Answer from the drawing. Dimensions are ordinates in mm from the lowest x, y and z of the part. A direction names the side the tool comes from. Coordinates: 2 decimals unless noted, no trailing zeros. Write each loop counter-clockwise with the first axis right and the second up, starting at its lowest first coordinate (ties: lowest second). Pieces come first, ordered by that corner, then holes. Notation, with made-up numbers: (72, -27.5) -> (127, -27.5) arc R14 cw to (127, -1.5) -> close; hole circle Ø5 at (-4.75, 2). An arc over 180 degrees is marked (long way). Answer as a JSON object with one key per item and string values. Group by question number.
(1) Flat-ended cylindrical pins translate along their axes: P1, Ø4.5, axis at y = 5, z = 5, coming from the -X side; P2, Ø4.5, axis at x = 23.5, z = 5.5, coming from the -Y side; P3, Ø3, axis at x = 20.5, z = 7, coming from the -Y side. Find the tip coordinate at first contact, or state that the pin passes through.
(2) Which of the six approach directions +Z, -Z, +X, -X, +Y, -Y give full straight-line access (tool end or side, diameter ignored) to the marked faces 1, 2, 3, 4 and 5?
(3) Find section D-D (x = 6.25). Give the vertices of the cut face in (y, z).
(4) Straight lines are drawn through the part: L1, parallel to Y at x = 43.75, z = 2; L2, parallel to X at y = 30.5, z = 1; L3, parallel to X at y = 68.75, z = 4. For each, find the intervals that lie inside material, in ascending order.
(5) Find section C-C (y = 15). Give the vertices of the cut face in (x, z).
(6) Find section B-B (y = 31.25). Give the vertices of the cut face in (x, z).
(7) Find section A-A (x = 24.5). Give the vertices of the cut face in (y, z).
(8) For a pull along Y with two mould halves and no side action, classify the marked faces 6, 7, 8 and 9 as +Y half, -Y half, draft (parallel to the pull), parting line (faces both ways), or undercut.
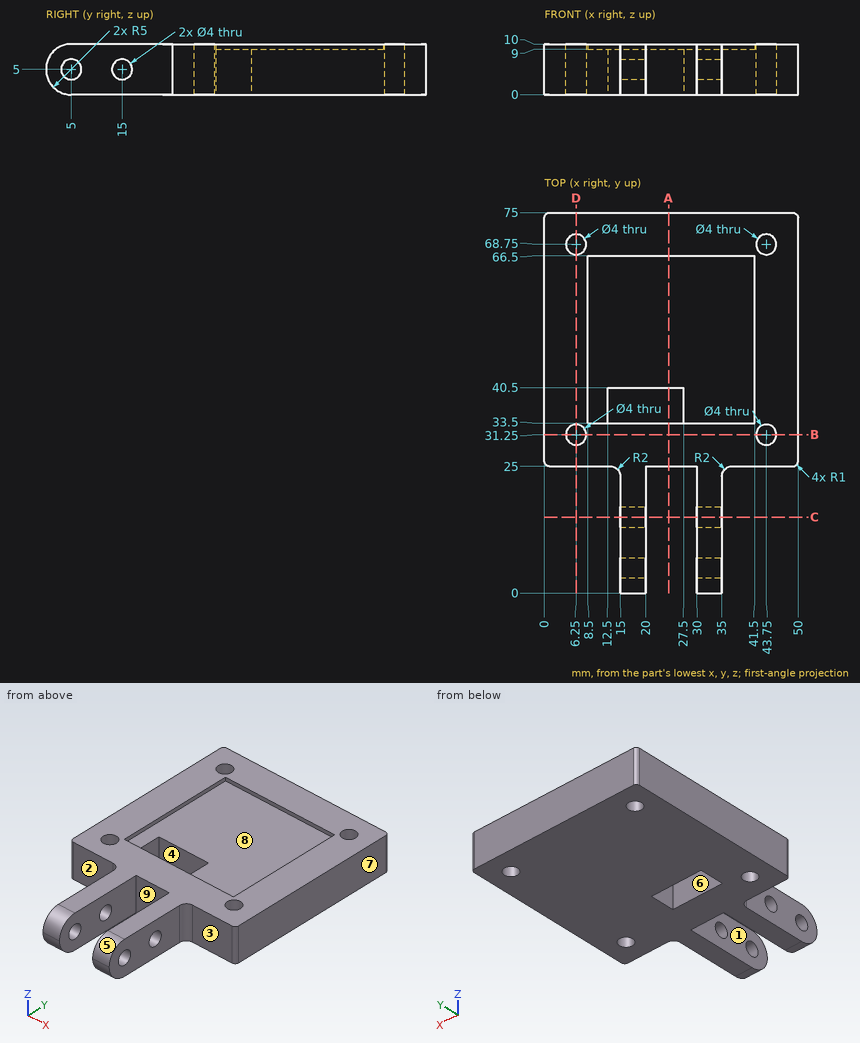
Results below:
{
 "1": {"P1": "stops at x = 15", "P2": "stops at y = 25", "P3": "stops at y = 0.03"},
 "2": {"face 1": "+Z, -Z, -Y", "face 2": "+Z, -Z, -X, -Y", "face 3": "+Z, -Z, +X, -Y", "face 4": "+Z, -Z", "face 5": "+Z, +X, -X, -Y"},
 "3": {"outline": "(25, 0) -> (29.25, 0) -> (29.25, 10) -> (25, 10) -> close; (33.25, 0) -> (66.75, 0) -> (66.75, 10) -> (33.25, 10) -> close; (70.75, 0) -> (75, 0) -> (75, 10) -> (70.75, 10) -> close"},
 "4": {"L1": "y = 25 to 29.25, 33.25 to 66.75, 70.75 to 75", "L2": "x = 0 to 4.4, 8.1 to 41.9, 45.6 to 50", "L3": "x = 0 to 4.25, 8.25 to 41.75, 45.75 to 50"},
 "5": {"outline": "(15, 0) -> (20, 0) -> (20, 3) -> (15, 3) -> close; (15, 7) -> (20, 7) -> (20, 10) -> (15, 10) -> close; (30, 0) -> (35, 0) -> (35, 3) -> (30, 3) -> close; (30, 7) -> (35, 7) -> (35, 10) -> (30, 10) -> close"},
 "6": {"outline": "(0, 0) -> (4.25, 0) -> (4.25, 10) -> (0, 10) -> close; (8.25, 0) -> (41.75, 0) -> (41.75, 10) -> (8.25, 10) -> close; (45.75, 0) -> (50, 0) -> (50, 10) -> (45.75, 10) -> close"},
 "7": {"outline": "(25, 0) -> (33.5, 0) -> (33.5, 10) -> (25, 10) -> close; (40.5, 0) -> (75, 0) -> (75, 10) -> (66.5, 10) -> (66.5, 9) -> (40.5, 9) -> close"},
 "8": {"face 6": "undercut", "face 7": "draft", "face 8": "undercut", "face 9": "-Y half"}
}
